For this review, use the dimensioned drawing (mm, ordinates from the lowest corner) and the shaded views. A direction names the side the tool comes from. Coordinates: 2 decimals unless noted, no trailing zeros. Loops run counter-clockwise (first coordinate to the right, second up) from the corner with the lowest first, then second, coordinate; pieces in that order, holes last. Notation, with made-up numbers: M 15.25,3 L 22.25,3 A20 ccw 22.25,23 Z; hole C 7,34.25 d8. An arc over 180 degrees is marked long. Use CSV: the item, a comma, the result in double quotes. Start each with the question number.
1. Draft analysis for pull direction X (two halves, no side actions). For the marked faces 1, 2 and 3, state which applies: +X half, -X half, draft (parallel to the pull), parting line (faces both ways), or undercut.
2. Tool access review of the marked faces 4, 5 and 6: name each direction out of +Z, -Z, +X, -X, +Y, -Y from which nothing blocks a thin tool from reaching the whole face with its end or side.
3. Add section B-B, the plane y = 11. Write out the cut boundary in (x, z) (1 decimal).
4. Add section D-D, the plane z = 3. Write out the cut boundary in (x, y) (1 decimal).
5. For L1, parallel to Z at x = 13, y = 13.5; L2, parallel to X at y = 16, z = 7.75 (1 decimal); L3, parallel to Z at x = 5, y = 19 (1 decimal), list the stretches that pass through material, from the lowest coordinate up.
6. Add section C-C, the plane x = 10. Write out the cut boundary in (y, z) (1 decimal), then the cut area to 3 significant figures.
7. Clearance check with flat-ended pins moving along their axes: P1, Ø3, axis at x = 3.05, y = 19.62, coming from the -Z side; P2, Ø3, axis at x = 12.5, z = 2, coming from the -Y side; P3, Ø12.5, axis at x = 19.62, y = 19.62, coming from the -Z side; P4, Ø6, axis at y = 34.5, z = 9.5, coming from the -X side. State where each tip first meets the part, or that it passes through.
8. Add section A-A, the plane x = 36. Write out the cut boundary in (y, z) (1 decimal).
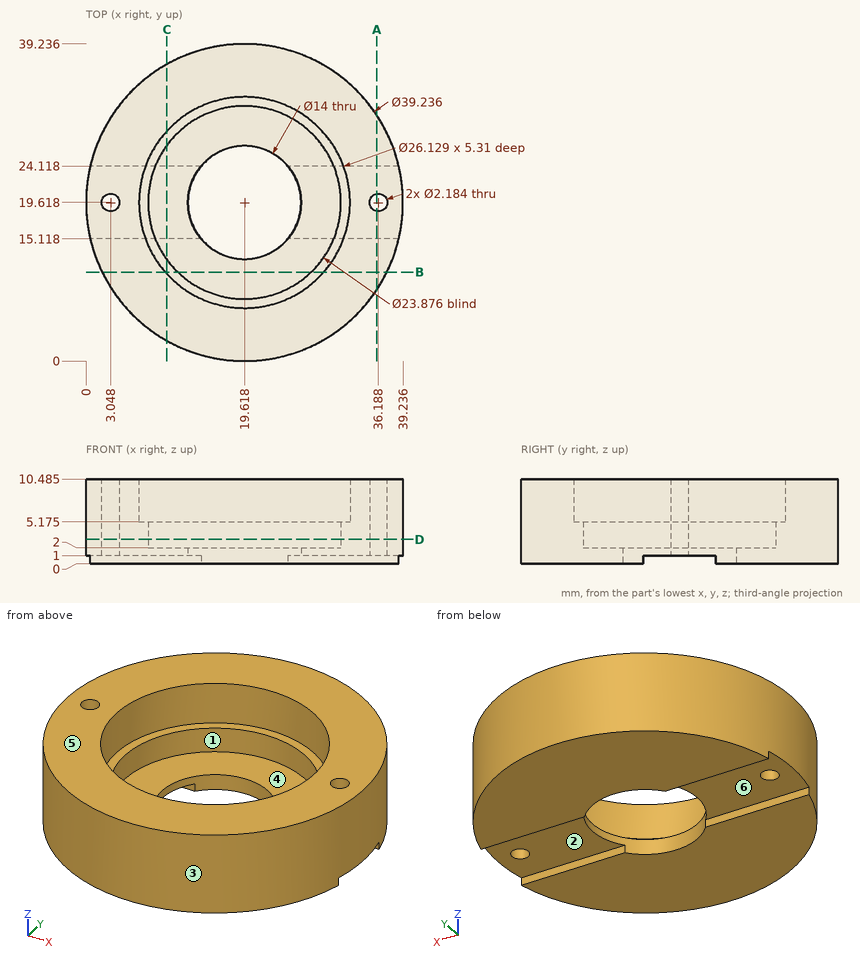
Computed:
1,face 1,"undercut"
1,face 2,"draft"
1,face 3,"parting line"
2,face 4,"+Z"
2,face 5,"+Z, +X, -X, +Y, -Y"
2,face 6,"-Z, +X, -X"
3,outline,"M 2,0 L 37.2,0 L 37.2,10.5 L 29.4,10.5 L 29.4,5.2 L 27.9,5.2 L 27.9,2 L 11.4,2 L 11.4,5.2 L 9.8,5.2 L 9.8,10.5 L 2,10.5 Z"
4,outline,"C 19.6,19.6 d39.2; hole C 3,19.6 d2.2; hole C 19.6,19.6 d23.9; hole C 36.2,19.6 d2.2"
5,L1,"z = 0 to 2"
5,L2,"x = 0.3 to 7.1, 32.2 to 38.9"
5,L3,"z = 1 to 10.5"
6,outline,"M 2.5,0 L 15.1,0 L 15.1,1 L 24.1,1 L 24.1,0 L 36.7,0 L 36.7,10.5 L 28.5,10.5 L 28.5,5.2 L 26.7,5.2 L 26.7,2 L 12.5,2 L 12.5,5.2 L 10.8,5.2 L 10.8,10.5 L 2.5,10.5 Z"
6,area,"211 mm^2"
7,P1,"stops at z = 1"
7,P2,"stops at y = 0.82"
7,P3,"passes through"
7,P4,"stops at x = 4.01"
8,outline,"M 8.8,0 L 15.1,0 L 15.1,1 L 18.5,1 L 18.5,10.5 L 8.8,10.5 Z; M 20.7,1 L 24.1,1 L 24.1,0 L 30.4,0 L 30.4,10.5 L 20.7,10.5 Z"
